The model under review builds one solid part; all positions refer to its coordinate system, in mm. Face numbers are marked on the shaded views. Round coordinates to 2 decimals unless told otherwise and drop trailing zeros. Order: outer loops, then holes, each group sorted by start corner. A loop starts at its lowest first (then second) coordinate and runs counter-clockwise, first axis right, second up. Notation, with made-up numbers: (-35.75, 6.5) -> (-3.75, 6.5) arc R20 cw to (-3.75, 27.5) -> close; hole circle Ø7 at (-1.5, 51). An arc over 180 degrees is marked (long way). Use a Markdown table: item, result. Add a question column.
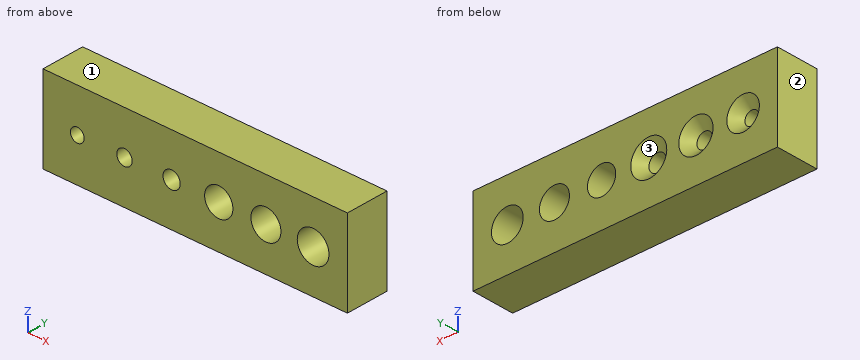
```python
from build123d import *

# Parameters (mm, degrees)
SKETCH1_W                             = 35.5
SKETCH1_H                             = 10
BOSS_EXTRUDE1_DEPTH                   = 5
TAP_DRILL_FOR_M2X0_4_TAP1_D           = 1.8
TAP_DRILL_FOR_M2X0_4_TAP1_DEPTH       = 7
TAP_DRILL_FOR_M2X0_4_TAP1_CSINK_D     = 4
TAP_DRILL_FOR_M2X0_4_TAP1_CSINK_ANGLE = 90
TAP_DRILL_FOR_M2X0_4_TAP1_TIP         = 0.540774557
TAP_DRILL_FOR_M2X0_4_TAP2_D           = 2
TAP_DRILL_FOR_M2X0_4_TAP2_DEPTH       = 7
TAP_DRILL_FOR_M2X0_4_TAP2_CSINK_D     = 4.2
TAP_DRILL_FOR_M2X0_4_TAP2_CSINK_ANGLE = 90
TAP_DRILL_FOR_M2X0_4_TAP2_TIP         = 0.600860619
TAP_DRILL_FOR_M2X0_4_TAP3_D           = 1.6
TAP_DRILL_FOR_M2X0_4_TAP3_DEPTH       = 7
TAP_DRILL_FOR_M2X0_4_TAP3_CSINK_D     = 3.8
TAP_DRILL_FOR_M2X0_4_TAP3_CSINK_ANGLE = 90
TAP_DRILL_FOR_M2X0_4_TAP3_TIP         = 0.480688495
TAP_DRILL_FOR_M4X0_7_TAP1_D           = 3.3
TAP_DRILL_FOR_M4X0_7_TAP1_DEPTH       = 5
TAP_DRILL_FOR_M4X0_7_TAP1_TIP         = 0.991420021
TAP_DRILL_FOR_M4X0_7_TAP2_D           = 3.5
TAP_DRILL_FOR_M4X0_7_TAP2_DEPTH       = 5
TAP_DRILL_FOR_M4X0_7_TAP2_TIP         = 1.051506083
TAP_DRILL_FOR_M4X0_7_TAP3_D           = 3.7
TAP_DRILL_FOR_M4X0_7_TAP3_DEPTH       = 5
TAP_DRILL_FOR_M4X0_7_TAP3_TIP         = 1.111592145


with BuildPart() as part:
    # Sketch1 → Boss-Extrude1 (new body)
    with BuildSketch(Plane(origin=(0, 0, 0), x_dir=(1, 0, 0), z_dir=(0, 1, 0))):
        with Locations((17.75, 5)):
            Rectangle(SKETCH1_W, SKETCH1_H)
    extrude(amount=BOSS_EXTRUDE1_DEPTH)

    # Tap Drill for M2x0.4 Tap1
    with Locations(Plane(origin=(9.5, 5, -5), x_dir=(0, 0, 1), z_dir=(0, 1, 0))):
        with Locations((0, 0)):
            CounterSinkHole(TAP_DRILL_FOR_M2X0_4_TAP1_D / 2, TAP_DRILL_FOR_M2X0_4_TAP1_CSINK_D / 2, depth=TAP_DRILL_FOR_M2X0_4_TAP1_DEPTH, counter_sink_angle=TAP_DRILL_FOR_M2X0_4_TAP1_CSINK_ANGLE)
            with Locations((0, 0, -(TAP_DRILL_FOR_M2X0_4_TAP1_DEPTH + TAP_DRILL_FOR_M2X0_4_TAP1_TIP / 2))):  # 118° drill point
                Cone(0, TAP_DRILL_FOR_M2X0_4_TAP1_D / 2, TAP_DRILL_FOR_M2X0_4_TAP1_TIP, mode=Mode.SUBTRACT)

    # Tap Drill for M2x0.4 Tap2
    with Locations(Plane(origin=(15, 5, -5), x_dir=(0, 0, 1), z_dir=(0, 1, 0))):
        with Locations((0, 0)):
            CounterSinkHole(TAP_DRILL_FOR_M2X0_4_TAP2_D / 2, TAP_DRILL_FOR_M2X0_4_TAP2_CSINK_D / 2, depth=TAP_DRILL_FOR_M2X0_4_TAP2_DEPTH, counter_sink_angle=TAP_DRILL_FOR_M2X0_4_TAP2_CSINK_ANGLE)
            with Locations((0, 0, -(TAP_DRILL_FOR_M2X0_4_TAP2_DEPTH + TAP_DRILL_FOR_M2X0_4_TAP2_TIP / 2))):  # 118° drill point
                Cone(0, TAP_DRILL_FOR_M2X0_4_TAP2_D / 2, TAP_DRILL_FOR_M2X0_4_TAP2_TIP, mode=Mode.SUBTRACT)

    # Tap Drill for M2x0.4 Tap3
    with Locations(Plane(origin=(4, 5, -5), x_dir=(0, 0, 1), z_dir=(0, 1, 0))):
        with Locations((0, 0)):
            CounterSinkHole(TAP_DRILL_FOR_M2X0_4_TAP3_D / 2, TAP_DRILL_FOR_M2X0_4_TAP3_CSINK_D / 2, depth=TAP_DRILL_FOR_M2X0_4_TAP3_DEPTH, counter_sink_angle=TAP_DRILL_FOR_M2X0_4_TAP3_CSINK_ANGLE)
            with Locations((0, 0, -(TAP_DRILL_FOR_M2X0_4_TAP3_DEPTH + TAP_DRILL_FOR_M2X0_4_TAP3_TIP / 2))):  # 118° drill point
                Cone(0, TAP_DRILL_FOR_M2X0_4_TAP3_D / 2, TAP_DRILL_FOR_M2X0_4_TAP3_TIP, mode=Mode.SUBTRACT)

    # Tap Drill for M4x0.7 Tap1
    with Locations(Plane(origin=(20.5, 5, -5), x_dir=(0, 0, 1), z_dir=(0, 1, 0))):
        with Locations((0, 0)):
            Hole(TAP_DRILL_FOR_M4X0_7_TAP1_D / 2, depth=TAP_DRILL_FOR_M4X0_7_TAP1_DEPTH)
            with Locations((0, 0, -(TAP_DRILL_FOR_M4X0_7_TAP1_DEPTH + TAP_DRILL_FOR_M4X0_7_TAP1_TIP / 2))):  # 118° drill point
                Cone(0, TAP_DRILL_FOR_M4X0_7_TAP1_D / 2, TAP_DRILL_FOR_M4X0_7_TAP1_TIP, mode=Mode.SUBTRACT)

    # Tap Drill for M4x0.7 Tap2
    with Locations(Plane(origin=(26, 5, -5), x_dir=(0, 0, 1), z_dir=(0, 1, 0))):
        with Locations((0, 0)):
            Hole(TAP_DRILL_FOR_M4X0_7_TAP2_D / 2, depth=TAP_DRILL_FOR_M4X0_7_TAP2_DEPTH)
            with Locations((0, 0, -(TAP_DRILL_FOR_M4X0_7_TAP2_DEPTH + TAP_DRILL_FOR_M4X0_7_TAP2_TIP / 2))):  # 118° drill point
                Cone(0, TAP_DRILL_FOR_M4X0_7_TAP2_D / 2, TAP_DRILL_FOR_M4X0_7_TAP2_TIP, mode=Mode.SUBTRACT)

    # Tap Drill for M4x0.7 Tap3
    with Locations(Plane(origin=(31.5, 5, -5), x_dir=(0, 0, 1), z_dir=(0, 1, 0))):
        with Locations((0, 0)):
            Hole(TAP_DRILL_FOR_M4X0_7_TAP3_D / 2, depth=TAP_DRILL_FOR_M4X0_7_TAP3_DEPTH)
            with Locations((0, 0, -(TAP_DRILL_FOR_M4X0_7_TAP3_DEPTH + TAP_DRILL_FOR_M4X0_7_TAP3_TIP / 2))):  # 118° drill point
                Cone(0, TAP_DRILL_FOR_M4X0_7_TAP3_D / 2, TAP_DRILL_FOR_M4X0_7_TAP3_TIP, mode=Mode.SUBTRACT)


solid = part.part
```
Q1. For pin 1 (2 mm diameter, centred on x = 31.5, z = -5, fed in from -Y); pin 2 (1 mm diameter, centred on x = 16.5, z = -5, fed in from +Y); pin 3 (3 mm diameter, centred on x = 9.5, z = -5, fed in from +Y), all flat-tipped, find the tip position at first contact; note any pin that passes through.
Q2. Draft analysis for pull direction Z (two halves, no side actions). For the marked faces 1, 2 and 3, state which applies: released by +Z, released by -Z, zero draft, split by the parting line, or undercut.
Q3. Add section D-D, the plane x = 26. Give the boundary of the cut face in (y, z).
Q4. Add section A-A, the plane x = 4. Give the boundary of the cut face in (y, z), then the cut area to 3 significant figures.
Q5. Add section C-C, the plane y = 4.4. Give the boundary of the cut face in (x, z).
Q6. Add section B-B, the plane z = -5. Give the number of separate pieces and of enclosed holes in the cut face, then the cut area to 3 significant figures.
Q7. To check wall thickness, follow line 1 along Z through (x, y) = (31.5, 3.6); line 2 along Z through (x, y) = (26, 2.15). State the ranges of each line that lie inside material, in increasing order.
Return value:
| question | item | result |
|---|---|---|
| 1 | pin 1 | through |
| 1 | pin 2 | y = 4.9 |
| 1 | pin 3 | y = 4.5 |
| 2 | face 1 | released by +Z |
| 2 | face 2 | zero draft |
| 2 | face 3 | undercut |
| 3 | outline | (0, -10) -> (5, -10) -> (5, -6.75) -> (0, -6.75) -> close; (0, -3.25) -> (5, -3.25) -> (5, 0) -> (0, 0) -> close |
| 4 | outline | (0, -10) -> (5, -10) -> (5, -6.9) -> (3.9, -5.8) -> (0, -5.8) -> close; (0, -4.2) -> (3.9, -4.2) -> (5, -3.1) -> (5, 0) -> (0, 0) -> close |
| 4 | area | 40.8 mm² |
| 5 | outline | (0, -10) -> (35.5, -10) -> (35.5, 0) -> (0, 0) -> close; hole circle Ø2.6 at (4, -5); hole circle Ø2.8 at (9.5, -5); hole circle Ø3 at (15, -5); hole circle Ø3.3 at (20.5, -5); hole circle Ø3.5 at (26, -5); hole circle Ø3.7 at (31.5, -5) |
| 6 | separate pieces | 7 |
| 6 | enclosed holes | 0 |
| 6 | area | 94.4 mm² |
| 7 | line 1 | -10 to -6.85, -3.15 to 0 |
| 7 | line 2 | -10 to -6.75, -3.25 to 0 |
